Part model, mm, in its own coordinate system. A direction names the side the tool comes from. Give positions to 0.01 mm unless a question says otherwise; leave off trailing zeros. Order: outer loops, then holes, each group sorted by start corner. A loop starts at its lowest first (then second) coordinate and runs counter-clockwise, first axis right, second up. Notation, with made-up numbers: M 12,29.5 L 52,29.5 A19 cw 52,43.5 Z; hole C 59.25,76.5 d1. An arc over 180 degrees is marked long. One line per question, with ' | ' between items.
```python
from build123d import *

# Parameters (mm, degrees)
SKETCH_1_W          = 28
SKETCH_1_H          = 17
EXTRUDE_1_DEPTH     = 3
EXTRUDE_2_DEPTH     = 5.5
CUT_EXTRUDE_1_DEPTH = 2.5
RIB_4_REACH         = 22.304
SKETCH_5_WALL_W     = 57.313322178
SKETCH_5_WALL_H     = 3
FILLET_1_R          = 3
SKETCH_6_R          = 1.5
CUT_EXTRUDE_2_DEPTH = 5.3
EXTRUDE_3_DEPTH     = 5.5
CUT_EXTRUDE_3_DEPTH = 2.5
FILLET_3_R          = 3
FILLET_4_R          = 10


with BuildPart() as part:
    # 草图1 → 凸台-拉伸1 (new body)
    with BuildSketch(Plane.XY):
        Rectangle(SKETCH_1_W, SKETCH_1_H)
    extrude(amount=EXTRUDE_1_DEPTH)

    # 草图3 → 凸台-拉伸2 (add, symmetric)
    with BuildSketch(Plane(origin=(0, 0, 0), x_dir=(0, 0, -1), z_dir=(1, 0, 0))):
        Polygon((0, 8.5), (12, 1.57179677), (12, -6.5), (0, -6.5), (0, 1.57179677), align=None)
    extrude(amount=EXTRUDE_2_DEPTH, both=True)

    # 草图4 → 切除-拉伸1 (cut, symmetric)
    with BuildSketch(Plane(origin=(0, 0, 0), x_dir=(0, 0, -1), z_dir=(1, 0, 0))):
        Polygon((0, 8.5), (12, 1.57179677), (12, -3.160254038), (0, 3.767949192), (-3, 5.5), (-3, 10.232050808), align=None)
    extrude(amount=CUT_EXTRUDE_1_DEPTH, both=True, mode=Mode.SUBTRACT)

    # 草图5 wall → 筋4 (add, up to next)
    with BuildSketch(Plane(origin=(9.75, 0, -6), x_dir=(0.57801734078, 0, 0.816024481102), z_dir=(0.816024481102, 0, -0.57801734078)), mode=Mode.PRIVATE) as rib_4_sk1:
        Rectangle(SKETCH_5_WALL_W, SKETCH_5_WALL_H)
    rib_4_tool1 = extrude(rib_4_sk1.sketch, amount=-RIB_4_REACH, mode=Mode.PRIVATE) - part.part
    rib_4 = rib_4_tool1.solids().sort_by_distance((9.75, 0, -6))[0]
    add(rib_4)

    # 镜向1: 筋4 across plane
    add(rib_4.mirror(Plane(origin=(0, 0, 0), x_dir=(0, 0, 1), z_dir=(1, 0, 0))))

    # 圆角1
    fillet_1_edges = [part.edges().sort_by_distance(p)[0] for p in [
        (14, -8.5, 1.5),
        (-14, -8.5, 1.5),
        (-14, 8.5, 1.5),
        (14, 8.5, 1.5),
    ]]
    fillet(fillet_1_edges, radius=FILLET_1_R)

    # 草图6 → 切除-拉伸2 (cut)
    with BuildSketch(Plane(origin=(0, 0, 0), x_dir=(-1, 0, 0), z_dir=(0, 0, -1))):
        with Locations((-10.5, 5.5)):
            Circle(SKETCH_6_R)
        with Locations((10.5, 5.5)):
            Circle(SKETCH_6_R)
        with Locations((10.5, -5.5)):
            Circle(SKETCH_6_R)
        with Locations((-10.5, -5.5)):
            Circle(SKETCH_6_R)
    extrude(amount=-CUT_EXTRUDE_2_DEPTH, mode=Mode.SUBTRACT)

    # 草图7 → 凸台-拉伸3 (add, symmetric)
    with BuildSketch(Plane(origin=(0, 0, 0), x_dir=(0, 0, -1), z_dir=(1, 0, 0))):
        Polygon((0, 8.5), (12, 8.5), (12, 1.57179677), align=None)
    extrude(amount=EXTRUDE_3_DEPTH, both=True)

    # 草图7<2> → 切除-拉伸3 (cut, symmetric)
    with BuildSketch(Plane(origin=(0, 0, 0), x_dir=(0, 0, -1), z_dir=(1, 0, 0))):
        Polygon((0, 8.5), (12, 8.5), (12, 1.57179677), align=None)
    extrude(amount=CUT_EXTRUDE_3_DEPTH, both=True, mode=Mode.SUBTRACT)

    # 圆角3
    fillet_3_edges = [part.edges().sort_by_distance(p)[0] for p in [
        (4, 8.5, -12),
        (-4, 8.5, -12),
    ]]
    fillet(fillet_3_edges, radius=FILLET_3_R)

    # 圆角4
    # the kernel refuses this fillet: 10 mm, written as the material it takes off along each edge
    with BuildSketch(Plane(origin=(2.5, -3.160254038, -12), x_dir=(0, -1, 0), z_dir=(-1, 0, 0))) as fillet_4_piece_1:
        with BuildLine():
            CenterArc((FILLET_4_R * 0.57735026919, FILLET_4_R), FILLET_4_R, 210, 60)
            Line((-FILLET_4_R * 0.288675134595, FILLET_4_R * 0.5), (0, 0))
            Line((0, 0), (FILLET_4_R * 0.57735026919, 0))
        make_face()
    extrude(amount=5, mode=Mode.SUBTRACT)


solid = part.part
```
1. Tool access for faces 1 (the flat face through (8, 1.5, -3)), 2 (the flat face through (5.5, -4, -6)), 3 (the cylindrical face through (0.035, -2.865, -9.948)): list every direction of +Z, -Z, +X, -X, +Y, -Y with a clear straight run to the whole face (end or side of a thin tool).
Worked out:
face 1: -Z, +X, +Y | face 2: -Z, +X, -Y | face 3: -Z, +Y
2. Mould opens along X. For faces 4 (the flat face through (9.691, -0.021, -6.084)), 5 (the flat face through (0, 0, 3)), 6 (the cylindrical face through (-9, 5.57, 1.48)) say: released by +X, released by -X, zero draft, split by the parting line, or undercut.
Worked out:
face 4: released by +X | face 5: zero draft | face 6: undercut
3. Probe L1, parallel to Y at x = -10.5, z = 1.85; L2, parallel to X at y = 5.5, z = -1.5; L3, parallel to X at y = -6, z = -10.5. List the from-to ranges inside material, lowest first. Write a range as from..to.
Worked out:
L1: y = -8.5..-7, -4..4, 7..8.5 | L2: x = -5.5..-2.5, 2.5..5.5 | L3: x = -5.5..5.5
4. Slice it at A-A on y = 4.75. Give the cut face in (x, z).
Worked out:
outline: M -14,0 L -11.8,0 L -11.8,3 L -14,3 Z; M -9.2,0 L -5.5,0 L -5.5,-12 L -2.5,-12 L -2.5,1.7 L 2.5,1.7 L 2.5,-12 L 5.5,-12 L 5.5,0 L 9.2,0 L 9.2,3 L -9.2,3 Z; M 11.8,0 L 14,0 L 14,3 L 11.8,3 Z
5. Slice it at B-B on x = -10.5. Give the cut face in (y, z).
Worked out:
outline: M -8.5,0 L -7,0 L -7,3 L -8.5,3 Z; M -4,0 L -1.5,0 L -1.5,-4.94 L 1.5,-4.94 L 1.5,0 L 4,0 L 4,3 L -4,3 Z; M 7,0 L 8.5,0 L 8.5,3 L 7,3 Z
6. Slice it at D-D on x = -1. Give the cut face in (y, z), then the cut area to 3 significant figures.
Worked out:
outline: M -8.5,0 L -6.5,0 L -6.5,-11.7 A10 ccw -0.27,-7 L 5.5,3 L -8.5,3 Z | area: 116 mm2
7. Slice it at C-C on z = -6. Give the cut face in (x, y), then the cut area to 3 significant figures.
Worked out:
outline: M -9.75,-1.5 L -5.5,-1.5 L -5.5,-6.5 L 5.5,-6.5 L 5.5,-1.5 L 9.75,-1.5 L 9.75,1.5 L 5.5,1.5 L 5.5,8.5 L 2.5,8.5 L 2.5,0.3 L -2.5,0.3 L -2.5,8.5 L -5.5,8.5 L -5.5,1.5 L -9.75,1.5 Z | area: 150 mm2
8. Drop flat-ended pins along their axis: pin 1 (5 mm diameter, centred on y = -5.5, z = -5, fed in from -X); pin 2 (5.5 mm diameter, centred on y = 4.5, z = -4.5, fed in from +X); pin 3 (5.5 mm diameter, centred on x = 0, z = -4.5, fed in from -Y). Give the stop position or say it passes through.
Worked out:
pin 1: stops at x = -5.5 | pin 2: stops at x = 5.5 | pin 3: stops at y = -6.5
